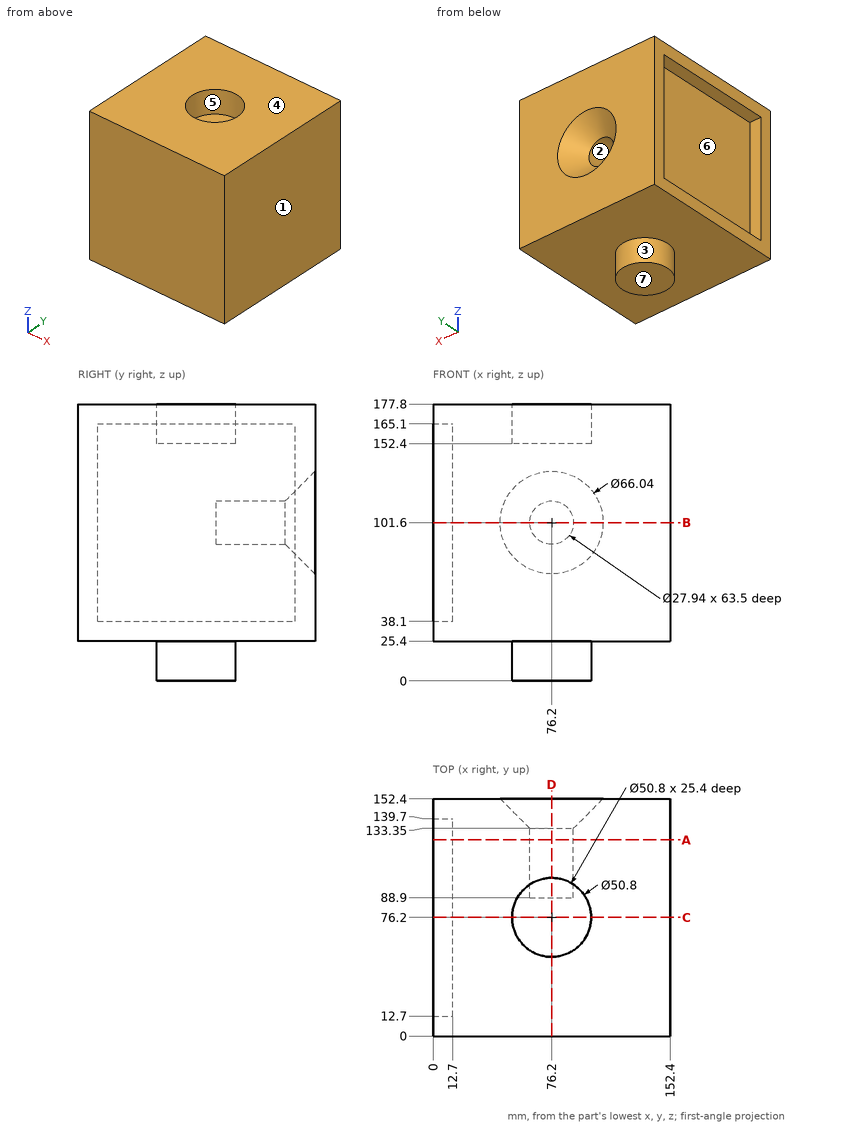
Geometry check sheet. Reference: drawing and pictorial views, mm from the part's lowest x, y, z. A direction names the side the tool comes from. Give positions to 0.01 mm unless a question says otherwise; leave off trailing zeros. Write each loop counter-clockwise with the first axis right and the second up, starting at its lowest first coordinate (ties: lowest second). Pieces come first, ordered by that corner, then holes.
Item 1: Access from +Z, -Z, +X, -X, +Y, -Y to the whole of each face (thin tool, end or side, straight path). Record for the marked faces 1, 2 and 3.
Item 2: Cross-section at B-B (z = 101.6). Enter the section's corners in (x, y).
Item 3: Cross-section at D-D (x = 76.2). Enter the section's corners in (y, z).
Item 4: Cross-section at C-C (y = 76.2). Enter the section's corners in (x, z).
Item 5: Scan lines: L1, parallel to Z at x = 76, y = 117; L2, parallel to X at y = 114, z = 101.6; L3, parallel to X at y = 95, z = 148. Record each from-to range of solid material in increasing order.
Item 6: Gauge pin test, flat ends, axial feed: pin 1 (14 mm diameter, centred on x = 70.5, z = 106.5, fed in from +Y); pin 2 (1.5 mm diameter, centred on x = 62.5, z = 95, fed in from -Y); pin 3 (8 mm diameter, centred on x = 48.5, y = 103.5, fed in from -Z); pin 4 (1 mm diameter, centred on x = 82.5, y = 68.5, fed in from +Z). Record the tip position at first contact, or that the pin passes through.
Item 7: Cross-section at A-A (y = 126). Enter the section's corners in (x, z).
Item 8: Draft check along Z on the marked faces 4, 5, 6 and 7. Enter one of: released by +Z, released by -Z, zero draft, split by the parting line, or undercut.
Report:
1. face 1: +Z, -Z, +X, +Y, -Y
1. face 2: +Y
1. face 3: -Z
2. outline: (0, 0) - (152.4, 0) - (152.4, 152.4) - (109.22, 152.4) - (90.17, 133.35) - (90.17, 88.9) - (62.23, 88.9) - (62.23, 133.35) - (43.18, 152.4) - (0, 152.4) - (0, 139.7) - (12.7, 139.7) - (12.7, 12.7) - (0, 12.7) - close
3. outline: (0, 25.4) - (50.8, 25.4) - (50.8, 0) - (101.6, 0) - (101.6, 25.4) - (152.4, 25.4) - (152.4, 68.58) - (133.35, 87.63) - (88.9, 87.63) - (88.9, 115.57) - (133.35, 115.57) - (152.4, 134.62) - (152.4, 177.8) - (101.6, 177.8) - (101.6, 152.4) - (50.8, 152.4) - (50.8, 177.8) - (0, 177.8) - close
4. outline: (0, 25.4) - (50.8, 25.4) - (50.8, 0) - (101.6, 0) - (101.6, 25.4) - (152.4, 25.4) - (152.4, 177.8) - (101.6, 177.8) - (101.6, 152.4) - (50.8, 152.4) - (50.8, 177.8) - (0, 177.8) - (0, 165.1) - (12.7, 165.1) - (12.7, 38.1) - (0, 38.1) - close
5. L1: z = 25.4 to 87.63, 115.57 to 177.8
5. L2: x = 12.7 to 62.23, 90.17 to 152.4
5. L3: x = 12.7 to 152.4
6. pin 1: stops at y = 133.9
6. pin 2: stops at y = 0
6. pin 3: stops at z = 25.4
6. pin 4: stops at z = 152.4
7. outline: (0, 25.4) - (152.4, 25.4) - (152.4, 177.8) - (0, 177.8) - (0, 165.1) - (12.7, 165.1) - (12.7, 38.1) - (0, 38.1) - close; hole circle Ø27.94 at (76.2, 101.6)
8. face 4: released by +Z
8. face 5: zero draft
8. face 6: undercut
8. face 7: released by -Z
